Print and shaded views of the part. All mm, measured from the part's lowest x, y and z. A direction names the side the tool comes from. Round coordinates to 2 decimals unless told otherwise and drop trailing zeros. Loops run counter-clockwise (first coordinate to the right, second up) from the corner with the lowest first, then second, coordinate; pieces in that order, holes last. Notation, with made-up numbers: (-34, 23.5) -> (-9, 23.5) arc R16 ccw to (-9, 40.5) -> close; hole circle Ø11 at (4.5, 73). An arc over 180 degrees is marked (long way). Answer as CSV lines item,"result".
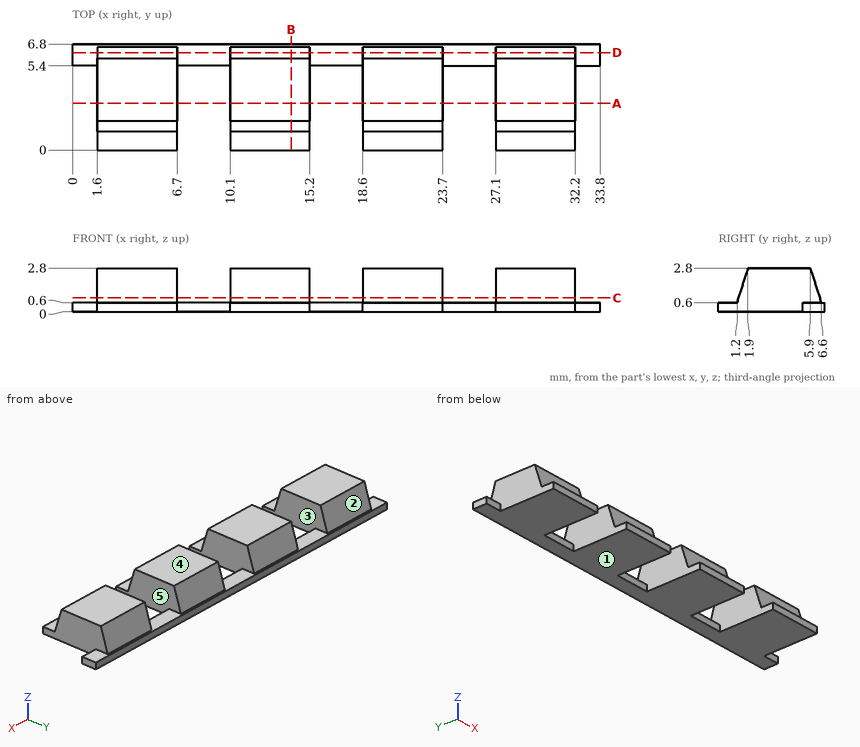
Q1. Slice it at B-B, the plane x = 14. Give the cut face in (y, z).
Results:
outline,"(0, 0) -> (6.8, 0) -> (6.8, 0.6) -> (6.6, 0.6) -> (5.9, 2.8) -> (1.9, 2.8) -> (1.2, 0.6) -> (0, 0.6) -> close"
Q2. Slice it at D-D, the plane y = 6.25. Give the cut face in (x, z), and give its area (3 significant figures).
Results:
outline,"(0, 0) -> (33.8, 0) -> (33.8, 0.6) -> (32.2, 0.6) -> (32.2, 1.7) -> (27.1, 1.7) -> (27.1, 0.6) -> (23.7, 0.6) -> (23.7, 1.7) -> (18.6, 1.7) -> (18.6, 0.6) -> (15.2, 0.6) -> (15.2, 1.7) -> (10.1, 1.7) -> (10.1, 0.6) -> (6.7, 0.6) -> (6.7, 1.7) -> (1.6, 1.7) -> (1.6, 0.6) -> (0, 0.6) -> close"
area,"42.7 mm2"
Q3. Tool access for the marked faces 4 and 5: list every direction of +Z, -Z, +X, -X, +Y, -Y with a clear straight run to the whole face (end or side of a thin tool).
Results:
face 4,"+Z, +X, -X, +Y, -Y"
face 5,"+Z, -Y"
Q4. Drop flat-ended pins along their axis: pin 1 Ø0.7 at (x, z) = (17, 0.5) entering from -Y; pin 2 Ø1 at (x, y) = (10, 2.5) entering from -Z; pin 3 Ø0.8 at (y, z) = (3.5, 1.5) entering from +X; pin 4 Ø0.8 at (y, z) = (3, 1) entering from -X. Give the stop position or say it passes through.
Results:
pin 1,"y = 5.4"
pin 2,"z = 0"
pin 3,"x = 32.2"
pin 4,"x = 1.6"
Q5. Two-plate mould, pull along Z, no slides. Class the marked faces 1, 2 and 3: pulls with the +Z half, pulls with the -Z half, needs draft (parallel to the pull), parting line crosses it, or undercut.
Results:
face 1,"pulls with the -Z half"
face 2,"pulls with the +Z half"
face 3,"needs draft"
Q6. Probe L1, parallel to X at y = 3.5, z = 2.05; L2, parallel to Z at x = 12, y = 0.5; L3, parallel to Y at x = 29, z = 2.75. List the from-to ranges inside material, lowest first. Write a range as [from, to].
Results:
L1,"[1.6, 6.7], [10.1, 15.2], [18.6, 23.7], [27.1, 32.2]"
L2,"[0, 0.6]"
L3,"[1.88, 5.92]"
Q7. Slice it at A-A, the plane y = 3. Give the cut face in (x, z).
Results:
outline,"(1.6, 0) -> (6.7, 0) -> (6.7, 2.8) -> (1.6, 2.8) -> close; (10.1, 0) -> (15.2, 0) -> (15.2, 2.8) -> (10.1, 2.8) -> close; (18.6, 0) -> (23.7, 0) -> (23.7, 2.8) -> (18.6, 2.8) -> close; (27.1, 0) -> (32.2, 0) -> (32.2, 2.8) -> (27.1, 2.8) -> close"
Q8. Slice it at C-C, the plane z = 0.9. Give the cut face in (x, y), and give its area (3 significant figures).
Results:
outline,"(1.6, 1.3) -> (6.7, 1.3) -> (6.7, 6.5) -> (1.6, 6.5) -> close; (10.1, 1.3) -> (15.2, 1.3) -> (15.2, 6.5) -> (10.1, 6.5) -> close; (18.6, 1.3) -> (23.7, 1.3) -> (23.7, 6.5) -> (18.6, 6.5) -> close; (27.1, 1.3) -> (32.2, 1.3) -> (32.2, 6.5) -> (27.1, 6.5) -> close"
area,"106 mm2"
